For this review, take the finished solid that the model builds, in its own axes (mm). Give positions to 0.01 mm unless a question says otherwise; leave off trailing zeros. Order: outer loops, then holes, each group sorted by start corner. A loop starts at its lowest first (then second) coordinate and runs counter-clockwise, first axis right, second up. Notation, with made-up numbers: M -31,34 L -8,34 A27 cw -8,51 Z; hole C 83,56 d5. An arc over 180 degrees is marked long. Use CSV: the item, a comma, the result in double quotes. Start each with the question number.
(1) Wall thickness on L1, parallel to Z at x = -13, y = -91; L2, parallel to X at y = -87.5, z = 30.5: over which ranges is each line inside the solid? List them lowest first. Write a range as from..to.
(2) Consider section A-A (x = -15.5). Write out the cut boundary in (y, z), and give its area (4 significant figures).
(3) Consider section B-B (y = -90.25). Write out the cut boundary in (x, z), and give its area (3 significant figures).
```python
from build123d import *

# Parameters (mm, degrees)
CROQUIS1_W              = 100
CROQUIS1_H              = 4
SALIENTE_EXTRUIR1_DEPTH = 37
CROQUIS2_W              = 100
CROQUIS2_H              = 37
SALIENTE_EXTRUIR2_DEPTH = 1
CROQUIS3_W              = 39
CROQUIS3_H              = 5.3
CORTAR_EXTRUIR1_DEPTH   = 10


with BuildPart() as part:
    # Croquis1 → Saliente-Extruir1 (new body)
    with BuildSketch(Plane.XY):
        with Locations((-0.047455137, -88.502540378)):
            Rectangle(CROQUIS1_W, CROQUIS1_H)
    extrude(amount=SALIENTE_EXTRUIR1_DEPTH)

    # Croquis2 → Saliente-Extruir2 (add)
    with BuildSketch(Plane.XZ.offset(90.502540378)):
        with Locations((-0.047455137, 18.5)):
            Rectangle(CROQUIS2_W, CROQUIS2_H)
    extrude(amount=SALIENTE_EXTRUIR2_DEPTH)

    # Croquis3 → Cortar-Extruir1 (cut)
    with BuildSketch(Plane.XZ.offset(91.502540378)):
        with Locations((-0.030380106, 30.774409531)):
            Rectangle(CROQUIS3_W, CROQUIS3_H)
    extrude(amount=-CORTAR_EXTRUIR1_DEPTH, mode=Mode.SUBTRACT)


solid = part.part
```
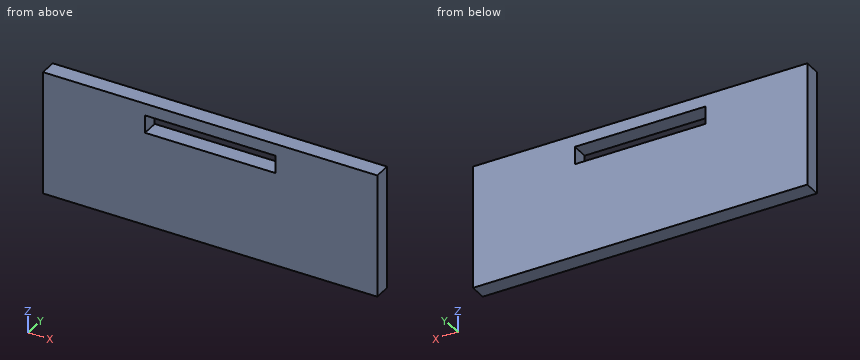
Check result:
1,L1,"z = 0..28.12, 33.42..37"
1,L2,"x = -50.05..-19.53, 19.47..49.95"
2,outline,"M -91.5,0 L -86.5,0 L -86.5,28.12 L -91.5,28.12 Z; M -91.5,33.42 L -86.5,33.42 L -86.5,37 L -91.5,37 Z"
2,area,"158.5 mm^2"
3,outline,"M -50.05,0 L 49.95,0 L 49.95,37 L -50.05,37 Z; hole M -19.53,28.12 L 19.47,28.12 L 19.47,33.42 L -19.53,33.42 Z"
3,area,"3,490 mm^2"
